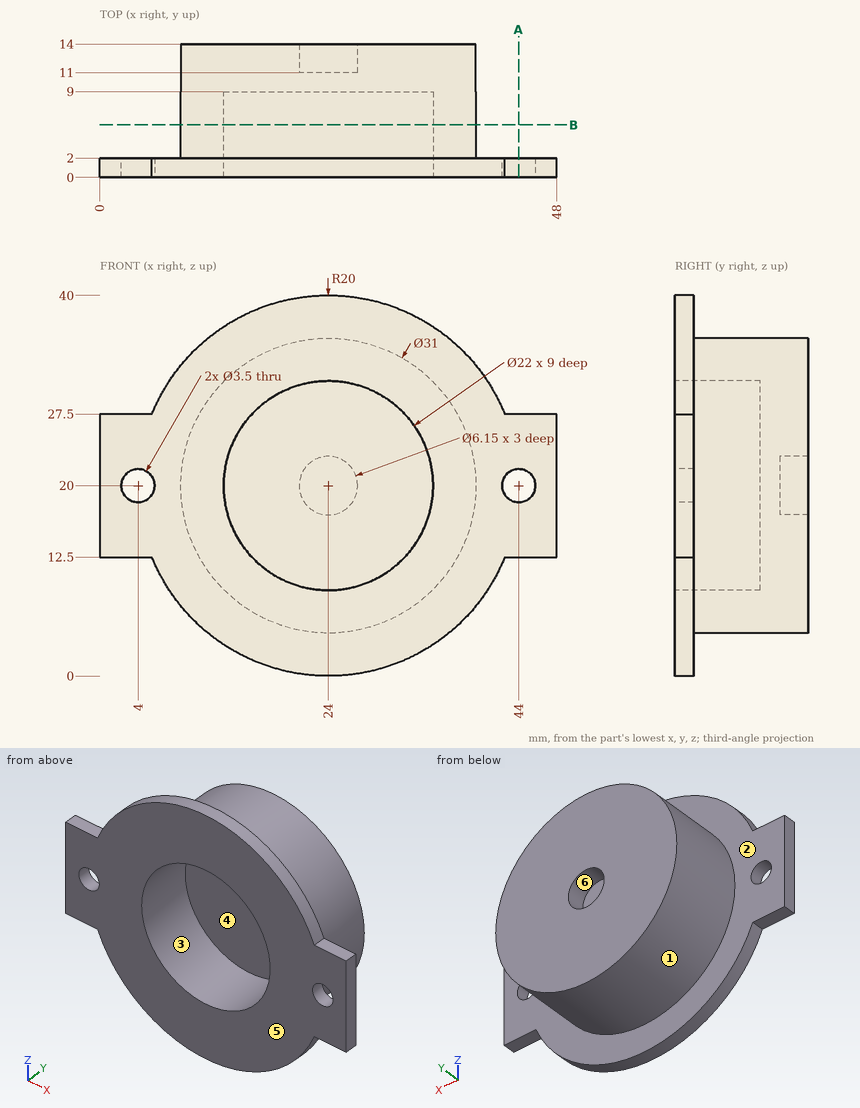
Print and shaded views of the part. All mm, measured from the part's lowest x, y and z. A direction names the side the tool comes from. Give positions to 0.01 mm unless a question says otherwise; leave off trailing zeros. Loops run counter-clockwise (first coordinate to the right, second up) from the corner with the lowest first, then second, coordinate; pieces in that order, holes last. Notation, with made-up numbers: (14, 18) - (55, 18) arc R28 cw to (55, 43) - close; hole circle Ø8 at (26, 68.5). An arc over 180 degrees is marked (long way). One line per item, written item: value. Start each with the question number.
1. Pull direction X, two halves, no side cores. Call the marked faces 1, 2 and 3: pulls with the +X half, pulls with the -X half, needs draft (parallel to the pull), parting line crosses it, or undercut.
2. Slice it at A-A (x = 44). List the corners of the cut face in (y, z).
3. Probe L1, parallel to X at y = 0.5, z = 20; L2, parallel to X at y = 5, z = 20; L3, parallel to X at y = 12.7, z = 20 (3 decimals). List the from-to ranges inside material, lowest first. Write a range as from..to.
4. Slice it at B-B (y = 5.5). List the corners of the cut face in (x, z).
5. Pin check, flat tips, straight feed: pin 1 (5 mm diameter, centred on x = 24, z = 20, fed in from -Y); pin 2 (0.6 mm diameter, centred on x = 2.5, y = 0.5, fed in from -Z); pin 3 (1.5 mm diameter, centred on x = 35, z = 5, fed in from -Y); pin 4 (3 mm diameter, centred on y = 8.5, z = 8, fed in from -X). Stop position of each tip, or through.
6. Which spindle directions (+Z, -Z, +X, -X, +Y, -Y) get a long thin tool onto all of the face, cutting with end or side? Do the marked faces 4, 5 and 6. Say none if no direction does.
Solution:
1. face 1: parting line crosses it
1. face 2: needs draft
1. face 3: undercut
2. outline: (0, 12.5) - (2, 12.5) - (2, 18.25) - (0, 18.25) - close; (0, 21.75) - (2, 21.75) - (2, 27.5) - (0, 27.5) - close
3. L1: x = 0..2.25, 5.75..13, 35..42.25, 45.75..48
3. L2: x = 8.5..13, 35..39.5
3. L3: x = 8.5..20.925, 27.075..39.5
4. outline: circle Ø31 at (24, 20); hole circle Ø22 at (24, 20)
5. pin 1: stops at y = 9
5. pin 2: stops at z = 12.5
5. pin 3: stops at y = 0
5. pin 4: stops at x = 12.6
6. face 4: -Y
6. face 5: +Z, -Z, +X, -X, -Y
6. face 6: +Y
